Could you check a few things on this drawing? It's one solid part, dimensions in mm from its lowest x, y, z. Coordinates: 2 decimals unless noted, no trailing zeros. Order: outer loops, then holes, each group sorted by start corner. A loop starts at its lowest first (then second) coordinate and runs counter-clockwise, first axis right, second up. Notation, with made-up numbers: (25, -36.75) - (32, -36.75) arc R13 cw to (32, -22.75) - close; hole circle Ø3 at (84, 70). An arc over 180 degrees is marked (long way). Answer in a Markdown table with one row per item. Add a question column.
Item 1: If I drill on line 1 along X through (y, z) = (18.25, 251); line 2 along X through (y, z) = (13.75, 250); line 3 along Z through (x, y) = (230.5, 14.5) (1 decimal), over which ranges is the centre line in solid material (lowest first)? Write a range as from..to.
Item 2: Will these pins go through, and if not, where does the flat tip stop? pin 1 Ø10 at (x, y) = (450, 9) entering from +Z (1 decimal); pin 2 Ø10 at (y, z) = (9.5, 398) entering from +X; pin 3 Ø6 at (y, z) = (6, 330) entering from +X.
Item 3: I want a section at A-A (y = 15.5). Count the separate pieces of the cut face and the enclosed holes in it, plus the area to 3 significant figures.
Item 4: I want a section at B-B (x = 250). Please give me the cut outline in (y, z).
Item 5: I want a section at C-C (z = 172.5). Please give me the cut outline in (x, y), plus the area to 3 significant figures.
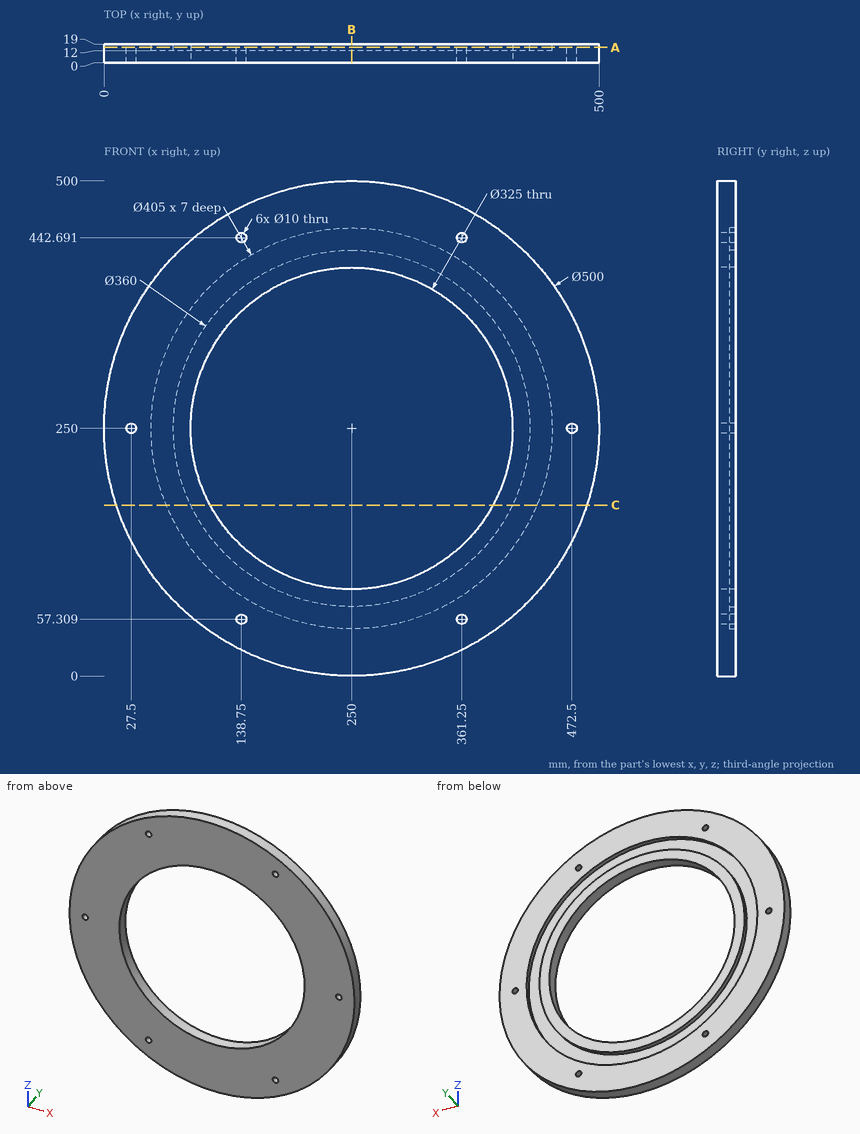
Values follow:
| question | item | result |
|---|---|---|
| 1 | line 1 | x = 0..22.6, 32.4..47.5, 70..87.5, 412.5..430, 452.5..467.6, 477.4..500 |
| 1 | line 2 | x = 0..22.5, 32.5..47.5, 70..87.5, 412.5..430, 452.5..467.5, 477.5..500 |
| 1 | line 3 | z = 0.8..48.4, 71.1..88.7, 411.3..428.9, 451.6..499.2 |
| 2 | pin 1 | stops at z = 406.4 |
| 2 | pin 2 | stops at x = 455.06 |
| 2 | pin 3 | stops at x = 487.85 |
| 3 | separate pieces | 2 |
| 3 | enclosed holes | 8 |
| 3 | area | 85,900 mm^2 |
| 4 | outline | (0, 0) - (19, 0) - (19, 47.5) - (12, 47.5) - (12, 70) - (19, 70) - (19, 87.5) - (0, 87.5) - close; (0, 412.5) - (19, 412.5) - (19, 430) - (12, 430) - (12, 452.5) - (19, 452.5) - (19, 500) - (0, 500) - close |
| 5 | outline | (12.32, 0) - (107.17, 0) - (107.17, 19) - (87.54, 19) - (87.54, 12) - (62.92, 12) - (62.92, 19) - (12.32, 19) - close; (392.83, 0) - (487.68, 0) - (487.68, 19) - (437.08, 19) - (437.08, 12) - (412.46, 12) - (412.46, 19) - (392.83, 19) - close |
| 5 | area | 3,260 mm^2 |
